from build123d import *

# Parameters (mm, degrees)
PAD005_DEPTH    = 1.6
SKETCH008_R     = 3.55
PAD006_DEPTH    = 15.6
SKETCH009_R     = 1.45
POCKET002_DEPTH = 12
POCKET003_DEPTH = 1.6


with BuildPart() as part:
    # Sketch007 → Pad005 (new body)
    with BuildSketch(Plane.XY):
        with BuildLine():
            Line((-59.5, 40.5), (59.5, 40.5))
            ThreePointArc((62.5, 37.5), (61.62132, 39.62132), (59.5, 40.5))
            Line((62.5, 37.5), (62.5, -37.5))
            ThreePointArc((59.5, -40.5), (61.62132, -39.62132), (62.5, -37.5))
            Line((59.5, -40.5), (-59.5, -40.5))
            ThreePointArc((-62.5, -37.5), (-61.62132, -39.62132), (-59.5, -40.5))
            Line((-62.5, -37.5), (-62.5, 37.5))
            ThreePointArc((-59.5, 40.5), (-61.62132, 39.62132), (-62.5, 37.5))
        make_face()
    extrude(amount=PAD005_DEPTH)

    # Sketch008 → Pad006 (join)
    with BuildSketch(Plane.XY):
        with Locations((-57.75, 35.75)):
            Circle(SKETCH008_R)
        with Locations((-17.75, 35.75)):
            Circle(SKETCH008_R)
        with Locations((17.75, 35.75)):
            Circle(SKETCH008_R)
        with Locations((57.75, 35.75)):
            Circle(SKETCH008_R)
        with Locations((57.75, -35.75)):
            Circle(SKETCH008_R)
        with Locations((17.75, -35.75)):
            Circle(SKETCH008_R)
        with Locations((-17.75, -35.75)):
            Circle(SKETCH008_R)
        with Locations((-57.75, -35.75)):
            Circle(SKETCH008_R)
    extrude(amount=PAD006_DEPTH)

    # Sketch009 (on DatumPlane) → Pocket002 (cut)
    with BuildSketch(Plane.XY.offset(15.6)):
        with Locations((-57.75, 35.75)):
            Circle(SKETCH009_R)
        with Locations((-17.75, 35.75)):
            Circle(SKETCH009_R)
        with Locations((17.75, 35.75)):
            Circle(SKETCH009_R)
        with Locations((57.75, 35.75)):
            Circle(SKETCH009_R)
        with Locations((-57.75, -35.75)):
            Circle(SKETCH009_R)
        with Locations((-17.75, -35.75)):
            Circle(SKETCH009_R)
        with Locations((17.75, -35.75)):
            Circle(SKETCH009_R)
        with Locations((57.75, -35.75)):
            Circle(SKETCH009_R)
    extrude(amount=-POCKET002_DEPTH, mode=Mode.SUBTRACT)

    # Sketch011 → Pocket003 (cut)
    with BuildSketch(Plane.XY):
        with BuildLine():
            ThreePointArc((-25, 5), (-30, 0), (-25, -5))
            Line((-25, -5), (25, -5))
            ThreePointArc((25, -5), (30, 0), (25, 5))
            Line((25, 5), (-25, 5))
        make_face()
    extrude(amount=POCKET003_DEPTH, mode=Mode.SUBTRACT)


with BuildPart() as part_1:
    # Body002 placement: moved
    add(part.part.moved(Location((0, 0, 76))))


solid = part_1.part
The model under review builds one solid part; all positions refer to its coordinate system, in mm. A direction names the side the tool comes from. Round coordinates to 2 decimals unless told otherwise and drop trailing zeros. Write each loop counter-clockwise with the first axis right and the second up, starting at its lowest first coordinate (ties: lowest second). Pieces come first, ordered by that corner, then holes. Notation, with made-up numbers: (31, 5) -> (52, 5) arc R28 ccw to (52, 29) -> close; hole circle Ø3 at (-19.5, -39). An arc over 180 degrees is marked (long way). Answer as a JSON object with one key per item and string values.
1. We need section A-A on z = 81. State how many separate pieces and enclosed holes the cut face has, and give its area (3 significant figures).
Results found:
{"separate pieces": "8", "enclosed holes": "8", "area": "264 mm^2"}
2. We need section C-C on x = -57.75. State the section outline as (y, z) points, and give its area (3 significant figures).
Results found:
{"outline": "(-40.5, 76) -> (40.5, 76) -> (40.5, 77.6) -> (39.3, 77.6) -> (39.3, 91.6) -> (37.2, 91.6) -> (37.2, 79.6) -> (34.3, 79.6) -> (34.3, 91.6) -> (32.2, 91.6) -> (32.2, 77.6) -> (-32.2, 77.6) -> (-32.2, 91.6) -> (-34.3, 91.6) -> (-34.3, 79.6) -> (-37.2, 79.6) -> (-37.2, 91.6) -> (-39.3, 91.6) -> (-39.3, 77.6) -> (-40.5, 77.6) -> close", "area": "259 mm^2"}
3. We need section D-D on y = -21. State the section outline as (x, z) points.
Results found:
{"outline": "(-62.5, 76) -> (62.5, 76) -> (62.5, 77.6) -> (-62.5, 77.6) -> close"}
4. To check wall thickness, follow line 1 along Y through (x, z) = (57.75, 84.25); line 2 along Z through (x, y) = (-6, -15); line 3 along X through (y, z) = (-2.5, 77.5). State the ranges of each line that lie inside material, in increasing order.
Results found:
{"line 1": "y = -39.3 to -37.2, -34.3 to -32.2, 32.2 to 34.3, 37.2 to 39.3", "line 2": "z = 76 to 77.6", "line 3": "x = -62.5 to -29.33, 29.33 to 62.5"}
5. We need section B-B on x = 9. State the section outline as (y, z) points.
Results found:
{"outline": "(-40.5, 76) -> (-5, 76) -> (-5, 77.6) -> (-40.5, 77.6) -> close; (5, 76) -> (40.5, 76) -> (40.5, 77.6) -> (5, 77.6) -> close"}
6. Machinability: for faces 1 (the face through (18.5, -37.3, 91.6)), 2 (the face through (61.03, 34.39, 84.5)), which of the approach directions +Z, -Z, +X, -X, +Y, -Y give a long, thin tool a straight path to every point of the face, cutting with its end or side? Answer none if there is none.
Results found:
{"face 1": "+Z, +X, -X, +Y, -Y", "face 2": "+Z"}
7. Clearance check with flat-ended pins moving along their axes: pin 1 (12 mm diameter, centred on x = 34.5, y = 6, fed in from +Z); pin 2 (2.5 mm diameter, centred on x = -17.75, y = 35.75, fed in from +Z); pin 3 (8 mm diameter, centred on y = 4.5, z = 85.5, fed in from -X). State where each tip first meets the part, or that it passes through.
Results found:
{"pin 1": "stops at z = 77.6", "pin 2": "stops at z = 79.6", "pin 3": "passes through"}
8. The part is to be moulded in two halves that separate along Y. For faces 3 (the face through (-16.411, 35.195, 85.684)), 4 (the face through (-61.64, -39.6, 76.79)), 5 (the face through (-18, 34, 91.6)), say which applies: pulls with the +Y half, pulls with the -Y half, needs draft (parallel to the pull), parting line crosses it, or undercut.
Results found:
{"face 3": "undercut", "face 4": "pulls with the -Y half", "face 5": "needs draft"}
